Can you work these out from the model? Positions are in its coordinate system, mm. A direction names the side the tool comes from. Give positions to 0.01 mm unless a question says otherwise; leave off trailing zeros. Order: outer loops, then holes, each group sorted by start corner. A loop starts at its lowest first (then second) coordinate and runs counter-clockwise, first axis right, second up. Notation, with made-up numbers: M 34,4.5 L 66,4.5 A8 ccw 66,16.5 Z; hole C 41.5,55.25 d5. An arc over 180 degrees is marked long. Use a Markdown table: item, result. Add a question column.
Autodesk Inventor part; units mm, degrees
ref_plane "YZ Plane" through (0, 0, 0) normal (1, 0, 0) x (0, 1, 0)
ref_plane "XZ Plane" through (0, 0, 0) normal (0, 1, 0) x (-1, 0, 0)
ref_plane "XY Plane" through (0, 0, 0) normal (0, 0, 1) x (1, 0, 0)
sketch "Sketch1" plane through (0, 0, 0) normal (0, 1, 0) x (-1, 0, 0)
  line L0 (0, 0) -> (-50.8, 0)
  line L1 (-50.8, 0) -> (-50.8, -76.2)
  line L2 (-50.8, -76.2) -> (0, -76.2)
  line L3 (0, -76.2) -> (0, 0)
  line L4 (-4.0754, 0) -> (-4.0754, -6.35)
  line L5 (0, -6.35) -> (-6.35, -6.35)
  line L6 (-50.8, -76.2) -> (-50.8, -69.85)
  line L7 (-50.8, -69.85) -> (-44.45, -69.85)
  line L8 (-6.35, -6.35) -> (-44.45, -6.35)
  line L9 (-44.45, -6.35) -> (-44.45, -69.85)
  line L10 (-44.45, -69.85) -> (-6.35, -69.85)
  line L11 (-6.35, -69.85) -> (-6.35, -6.35)
  dimension "d0" = 50.8
  dimension "d1" = 76.2
  dimension "d2" = 6.35
  dimension "d3" = 6.35
  dimension "d4" = 6.35
  dimension "d5" = 6.35
sketch "Sketch2" plane through (0, 0, 0) normal (0, 1, 0) x (-1, 0, 0)
  line L0 (-15.4991, -17.1025) -> (-35.8913, -17.1025)
  line L1 (-35.8913, -17.1025) -> (-35.8913, -58.0981)
  line L2 (-35.8913, -58.0981) -> (-15.4991, -58.0981)
  line L3 (-15.4991, -58.0981) -> (-15.4991, -17.1025)
  line L4 (-13.6908, -9.3345) -> (-8.6145, -9.1421)
  line L5 (-38.0829, -65.7666) -> (-42.7545, -67.7622)
  line L6 (-8.6145, -9.1421) -> (-42.7545, -9.1421)
  line L7 (-42.7545, -9.1421) -> (-42.7545, -67.7622)
  line L8 (-42.7545, -67.7622) -> (-8.6145, -67.7622)
  line L9 (-8.6145, -67.7622) -> (-8.6145, -9.1421)
  circle A0 centre (-20.5918, -13.1147) radius 1.651
  circle A1 centre (-30.7772, -13.1147) radius 1.651
  circle A2 centre (-20.5918, -62.0859) radius 1.651
  circle A3 centre (-30.7772, -62.0859) radius 1.651
  point P0 (0, 0)
  dimension "d6" = 40.9956
  dimension "d7" = 7.9756
  dimension "d8" = 5.08
  dimension "d9" = 7.9756
  dimension "d10" = 5.08
  dimension "d11" = 3.302
  dimension "d12" = 3.302
  dimension "d13" = 3.302
  dimension "d14" = 3.302
  dimension "d15" = 6.8846
  dimension "d16" = 6.8633
sketch "Sketch3" plane through (0, 0, 0) normal (0, 1, 0) x (-1, 0, 0)
  line L0 (-6.35, -6.35) -> (-44.45, -6.35)
  line L1 (-44.45, -6.35) -> (-44.45, -69.85)
  line L2 (-44.45, -69.85) -> (-6.35, -69.85)
  line L3 (-6.35, -69.85) -> (-6.35, -6.35)
  point P0 (0, 0)
extrude "Extrusion1" add sketch "Sketch1" along normal blind 76.2
sketch "Sketch4" plane through (0, 76.2, 0) normal (0, 1, 0) x (1, 0, 0)
  line L0 (45.1232, 71.603) -> (4.9996, 71.603)
  line L1 (4.9996, 71.603) -> (4.9996, 3.7205)
  line L2 (4.9996, 3.7205) -> (45.1232, 3.7205)
  line L3 (45.1232, 3.7205) -> (45.1232, 71.603)
  point P0 (0, 0)
extrude "Extrusion2" cut sketch "Sketch4" against normal blind 69.85
sketch "Sketch5" plane through (50.8, 0, -76.2) normal (0, 0, -1) x (-1, 0, 0)
  circle A0 centre (24.7613, 36.4788) radius 8.1657
  point P0 (50.8, 0)
extrude "Extrusion3" cut sketch "Sketch5" against normal blind 25.4
extrude "Extrusion4" cut sketch "Sketch2" along normal through all contours L3 L2 L1 L0 | A0 | A1 | A2 | A3
1. If we section it at A-A, the plane y = 19.5: List the corners of the cut face in (x, z) for me.
2. We'd pull the mould along X, two halves only. Please class faces 4 (the face through (21.649, 43.364, -73.934)), 5 (the face through (50.8, 38, -38)), 6 (the face through (26, 46, -76.2)): +X half, -X half, draft (parallel to the pull), parting line (faces both ways), or undercut.
3. If we section it at C-C, the plane x = 28: List the corners of the cut face in (y, z) for me.
4. I need wall thicknesses on L1, parallel to Z at x = 41, y = 19.5; L2, parallel to X at y = 62, z = -48; L3, parallel to Y at x = 11.5, z = -58. Which ranges of each line are inside material? Lowest first, please. Write a range as [from, to].
5. If we section it at B-B, the plane z = -32.5: List the corners of the cut face in (x, y) for me, then the cut area to 3 significant figures.
6. If we section it at D-D, the plane z = -68: List the corners of the cut face in (x, y) for me, then the cut area to 3 significant figures.
7. On a 3-axis mill with a long thin cutter (end or side, diameter ignored), from which of +Z, -Z, +X, -X, +Y, -Y can I reach the whole of each face in a straight line? I mean faces 1 (the face through (26, 3, -17.102)), 2 (the face through (5, 42, -38)), 3 (the face through (0, 38, -39)). Say none if no direction works.
8. Will these pins go through, and if not, where does the flat tip stop? pin 1 (3 mm diameter, centred on x = 20.59, z = -62.09, fed in from +Y); pin 2 (5.5 mm diameter, centred on x = 30.78, z = -62.09, fed in from +Y); pin 3 (10 mm diameter, centred on x = 26.04, y = 36.48, fed in from -Z).
Geometry results:
| question | item | result |
|---|---|---|
| 1 | outline | M 0,-76.2 L 50.8,-76.2 L 50.8,0 L 0,0 Z; hole M 5,-71.6 L 45.12,-71.6 L 45.12,-3.72 L 5,-3.72 Z |
| 2 | face 4 | undercut |
| 2 | face 5 | +X half |
| 2 | face 6 | draft |
| 3 | outline | M 0,-76.2 L 28.55,-76.2 L 28.55,-71.6 L 6.35,-71.6 L 6.35,-58.1 L 0,-58.1 Z; M 0,-17.1 L 6.35,-17.1 L 6.35,-3.72 L 76.2,-3.72 L 76.2,0 L 0,0 Z; M 44.41,-76.2 L 76.2,-76.2 L 76.2,-71.6 L 44.41,-71.6 Z |
| 4 | L1 | z = [-76.2, -71.6], [-3.72, 0] |
| 4 | L2 | x = [0, 5], [45.12, 50.8] |
| 4 | L3 | y = [0, 6.35] |
| 5 | outline | M 0,0 L 15.5,0 L 15.5,6.35 L 5,6.35 L 5,76.2 L 0,76.2 Z; M 35.89,0 L 50.8,0 L 50.8,76.2 L 45.12,76.2 L 45.12,6.35 L 35.89,6.35 Z |
| 5 | area | 939 mm^2 |
| 6 | outline | M 0,0 L 50.8,0 L 50.8,76.2 L 45.12,76.2 L 45.12,6.35 L 5,6.35 L 5,76.2 L 0,76.2 Z |
| 6 | area | 1,070 mm^2 |
| 7 | face 1 | +Y, -Y |
| 7 | face 2 | +Y |
| 7 | face 3 | +Z, -Z, -X, +Y, -Y |
| 8 | pin 1 | passes through |
| 8 | pin 2 | stops at y = 6.35 |
| 8 | pin 3 | stops at z = -3.72 |
